Build history of the part. All positions in model axes, mm. A direction names the side the tool comes from. Give positions to 0.01 mm unless a question says otherwise; leave off trailing zeros. Order: outer loops, then holes, each group sorted by start corner. A loop starts at its lowest first (then second) coordinate and runs counter-clockwise, first axis right, second up. Notation, with made-up numbers: (-25.5, -32) - (-19.5, -32) arc R15 cw to (-19.5, -13) - close; hole circle Ø9 at (35, -30). An arc over 180 degrees is marked (long way). Use a Markdown table: item, result. Add a question column.
(1) Mould opens along Z. For faces 1 (the face through (0, 127, 0)), 2 (the face through (0, 127, 50)), 3 (the face through (0, 207.5, 25)), 4 (the face through (-7.5, 123, 25)) say: +Z half, -Z half, draft (parallel to the pull), parting line (faces both ways), or undercut.
(2) Slice it at D-D (z = 27.5). Write the cut outline in (x, y), then the cut area to 3 significant figures.
(3) Slice it at A-A (y = 215.5). Write the cut outline in (x, z).
(4) Wall check: line 1 (Y direction, x = 0, z = 6.75); line 2 (Z direction, x = -6.25, y = 26); line 3 (Y direction, x = -2.25, z = 3). Give the ranges that are in metal, low to high.
(5) Slice it at C-C (z = 3). Write the cut outline in (x, y), then the cut area to 3 significant figures.
(6) Flat gauge pins, fed straight in: pin 1 (9 mm diameter, centred on x = 0, y = 0, fed in from -Z); pin 2 (7.5 mm diameter, centred on x = -1, z = 20.5, fed in from +Y); pin 3 (2 mm diameter, centred on x = -1, z = 34.5, fed in from -Y); pin 4 (6 mm diameter, centred on x = -5.5, z = 6.5, fed in from +Y). Where does each tip first touch, or does it go through?
(7) Which spindle directions (+Z, -Z, +X, -X, +Y, -Y) get a long thin tool onto all of the face, cutting with end or side? Do faces 5 (the face through (-0.16, 257.5, 43.66)), 6 (the face through (0, 232, 12.5)), 7 (the face through (0, 25, 12.5)). Say none if no direction does.
(8) Slice it at B-B (x = 0). Write the cut outline in (y, z), then the cut area to 4 significant figures.
from build123d import *

# Parameters (mm, degrees)
EXTRUDE_1_DEPTH     = 50
SKETCH_2_W          = 25
SKETCH_2_H          = 50
SKETCH_2_H_2        = 65
CUT_EXTRUDE_1_DEPTH = 263.737987356
SKETCH_3_R          = 5
CUT_EXTRUDE_2_DEPTH = 263.416653435


with BuildPart() as part:
    # 草图1 → 凸台-拉伸1 (new body)
    with BuildSketch(Plane.XY):
        with BuildLine():
            Line((-7.5, 0), (-7.5, 250))
            ThreePointArc((-7.5, 250), (0, 257.5), (7.5, 250))
            Line((7.5, 250), (7.5, 0))
            ThreePointArc((7.5, 0), (0, -7.5), (-7.5, 0))
        make_face()
    extrude(amount=EXTRUDE_1_DEPTH)

    # 草图2 → 切除-拉伸1 (cut, through all)
    with BuildSketch(Plane(origin=(7.5, 0, 0), x_dir=(0, 0, -1), z_dir=(1, 0, 0))):
        with Locations((-25, 232.5)):
            Rectangle(SKETCH_2_W, SKETCH_2_H)
        with Locations((-25, 25)):
            Rectangle(SKETCH_2_W, SKETCH_2_H_2)
    extrude(amount=-CUT_EXTRUDE_1_DEPTH, mode=Mode.SUBTRACT)

    # 草图3 → 切除-拉伸2 (cut, through all)
    with BuildSketch(Plane.XY.offset(50)):
        with Locations((0, 250)):
            Circle(SKETCH_3_R)
        Circle(SKETCH_3_R)
    extrude(amount=-CUT_EXTRUDE_2_DEPTH, mode=Mode.SUBTRACT)


solid = part.part
Solution:
| question | item | result |
|---|---|---|
| 1 | face 1 | -Z half |
| 1 | face 2 | +Z half |
| 1 | face 3 | undercut |
| 1 | face 4 | draft |
| 2 | outline | (-7.5, 57.5) - (7.5, 57.5) - (7.5, 207.5) - (-7.5, 207.5) - close |
| 2 | area | 2,250 mm2 |
| 3 | outline | (-7.5, 0) - (7.5, 0) - (7.5, 12.5) - (-7.5, 12.5) - close; (-7.5, 37.5) - (7.5, 37.5) - (7.5, 50) - (-7.5, 50) - close |
| 4 | line 1 | -7.5 to -5, 5 to 245, 255 to 257.5 |
| 4 | line 2 | 0 to 12.5, 37.5 to 50 |
| 4 | line 3 | -7.15 to -4.47, 4.47 to 245.53, 254.47 to 257.15 |
| 5 | outline | (-7.5, 0) arc R7.5 ccw to (7.5, 0) - (7.5, 250) arc R7.5 ccw to (-7.5, 250) - close; hole circle Ø10 at (0, 0); hole circle Ø10 at (0, 250) |
| 5 | area | 3,770 mm2 |
| 6 | pin 1 | through |
| 6 | pin 2 | y = 207.5 |
| 6 | pin 3 | y = 57.5 |
| 6 | pin 4 | y = 257.07 |
| 7 | face 5 | +Z, -Z, +Y |
| 7 | face 6 | +X, -X, +Y |
| 7 | face 7 | +X, -X, -Y |
| 8 | outline | (-7.5, 0) - (-5, 0) - (-5, 12.5) - (-7.5, 12.5) - close; (-7.5, 37.5) - (-5, 37.5) - (-5, 50) - (-7.5, 50) - close; (5, 0) - (245, 0) - (245, 12.5) - (207.5, 12.5) - (207.5, 37.5) - (245, 37.5) - (245, 50) - (5, 50) - (5, 37.5) - (57.5, 37.5) - (57.5, 12.5) - (5, 12.5) - close; (255, 0) - (257.5, 0) - (257.5, 12.5) - (255, 12.5) - close; (255, 37.5) - (257.5, 37.5) - (257.5, 50) - (255, 50) - close |
| 8 | area | 9,875 mm2 |
